Read the model definition and answer for the solid it produces. Units are mm, in the model's axes. Face numbers are marked on the shaded views. A direction names the side the tool comes from. Give positions to 0.01 mm unless a question says otherwise; leave off trailing zeros. Loops run counter-clockwise (first coordinate to the right, second up) from the corner with the lowest first, then second, coordinate; pieces in that order, holes last.
(1) Find section C-C, the plane x = 64.5. Write down the section's boundary in (y, z).
(2) Find section D-D, the plane z = -62.5. Write down the section's boundary in (x, y), then the cut area to 3 significant figures.
(3) Which of the six approach directions +Z, -Z, +X, -X, +Y, -Y give full straight-line access (tool end or side, diameter ignored) to the marked faces 1, 2 and 3?
(4) Find section B-B, the plane z = -46.56. Write down the section's boundary in (x, y), then the cut area to 3 significant figures.
(5) Find section A-A, the plane x = 13.54. Write down the section's boundary in (y, z).
(6) Straight lines are drawn through the part: probe 1 along Z at (x, y) = (128.95, 3.4); probe 2 along Z at (x, y) = (134.03, 3.3); probe 3 along X at (y, z) = (18.25, -23.5). For each, find the intervals that lie inside material, in ascending order.
(7) Each of these flat-tipped pins is pushed along its axis until it touches: P1, Ø7, axis at x = 113.71, z = -66.88, coming from the +Y side; P2, Ø10, axis at x = 36.5, y = 21, coming from the -Z side; P3, Ø7.5, axis at y = 18.5, z = -40.5, coming from the +X side. Where does it stop, or does it pass through?
(8) Determine the mould class of the marked faces 4, 5 and 6 for opening direction Z: pulls with the +Z half, pulls with the -Z half, needs draft (parallel to the pull), parting line crosses it, or undercut.
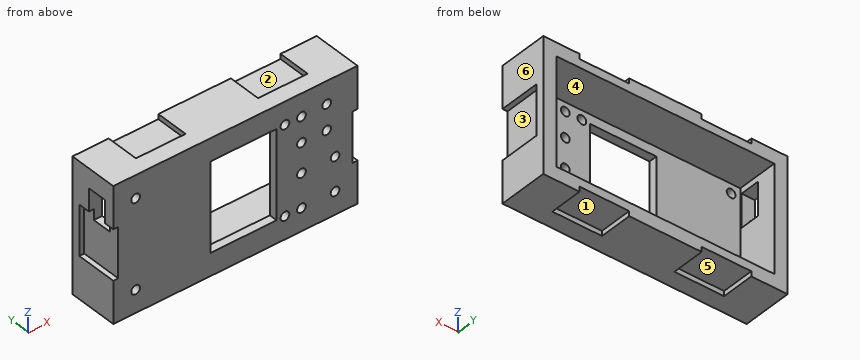
```python
from build123d import *

# Parameters (mm, degrees)
SKETCH1_W                  = 147.57
SKETCH1_H                  = 80.42
BOSS_EXTRUDE1_DEPTH        = 30
SKETCH2_W                  = 131.57
SKETCH2_H                  = 64.42
CUT_EXTRUDE1_DEPTH         = 25
F_4_0_209_DIAMETER_HOLE1_D = 5.3086
SKETCH13_W                 = 30
SKETCH13_H                 = 20
CUT_EXTRUDE3_DEPTH         = 3
MIRROR3_COPY_1_SKETCH_W    = 30
MIRROR3_COPY_1_SKETCH_H    = 20
MIRROR3_COPY_1_DEPTH       = 3
SKETCH19_W                 = 30
SKETCH19_H                 = 25
CUT_EXTRUDE4_DEPTH         = 3
SKETCH25_W                 = 40
SKETCH25_H                 = 53.34
CUT_EXTRUDE5_DEPTH         = 170.909626861
SKETCH30_W                 = 20
SKETCH30_H                 = 12
CUT_EXTRUDE7_DEPTH         = 164.851033869


with BuildPart() as part:
    # Sketch1 → Boss-Extrude1 (new body)
    with BuildSketch(Plane(origin=(0, 0, 0), x_dir=(1, 0, 0), z_dir=(0, 1, 0))):
        with Locations((73.785, 40.21)):
            Rectangle(SKETCH1_W, SKETCH1_H)
    extrude(amount=BOSS_EXTRUDE1_DEPTH)

    # Sketch2 → Cut-Extrude1 (cut)
    with BuildSketch(Plane(origin=(0, 30, 0), x_dir=(1, 0, 0), z_dir=(0, 1, 0))):
        with Locations((73.785, 40.21)):
            Rectangle(SKETCH2_W, SKETCH2_H)
    extrude(amount=-CUT_EXTRUDE1_DEPTH, mode=Mode.SUBTRACT)

    # #4 (0.209) Diameter Hole1 (through all)
    with Locations(Plane(origin=(13.54, 5, -66.88), x_dir=(0, 0, 1), z_dir=(0, 1, 0))):
        with Locations((0, 0), (53.34, 0), (53.34, 90.17), (53.34, 100.17), (38.1, 100.17), (38.1, 115.41), (53.34, 115.41), (20.32, 120.49), (0, 120.49), (0, 100.17), (20.32, 100.17), (0, 90.17)):
            Hole(F_4_0_209_DIAMETER_HOLE1_D / 2)

    # Sketch13 → Cut-Extrude3 (cut)
    with BuildSketch(Plane(origin=(0, 0, -80.42), x_dir=(-1, 0, 0), z_dir=(0, 0, -1))):
        with Locations((-110.6775, 20)):
            Rectangle(SKETCH13_W, SKETCH13_H)
    cut_extrude3 = extrude(amount=-CUT_EXTRUDE3_DEPTH, mode=Mode.SUBTRACT)

    # Mirror2: Cut-Extrude3 across plane
    add(cut_extrude3.mirror(Plane(origin=(73.785, 0, 0), x_dir=(0, 0, 1), z_dir=(1, 0, 0))), mode=Mode.SUBTRACT)

    # Mirror3: Cut-Extrude3 across plane
    add(cut_extrude3.mirror(Plane(origin=(0, 0, -40.21), x_dir=(1, 0, 0), z_dir=(0, 0, -1))), mode=Mode.SUBTRACT)

    # Mirror3 copy 1 sketch → Mirror3 copy 1 (cut)
    with BuildSketch(Plane(origin=(147.57, 0, 0), x_dir=(1, 0, 0), z_dir=(0, 0, 1))):
        with Locations((-110.6775, 20)):
            Rectangle(MIRROR3_COPY_1_SKETCH_W, MIRROR3_COPY_1_SKETCH_H)
    extrude(amount=-MIRROR3_COPY_1_DEPTH, mode=Mode.SUBTRACT)

    # Sketch19 → Cut-Extrude4 (cut)
    with BuildSketch(Plane.ZY):
        with Locations((-40.21, 12.5)):
            Rectangle(SKETCH19_W, SKETCH19_H)
    cut_extrude4 = extrude(amount=-CUT_EXTRUDE4_DEPTH, mode=Mode.SUBTRACT)

    # Mirror7: Cut-Extrude4 across plane
    add(cut_extrude4.mirror(Plane(origin=(73.785, 0, 0), x_dir=(0, 0, 1), z_dir=(1, 0, 0))), mode=Mode.SUBTRACT)

    # Sketch25 → Cut-Extrude5 (cut, through all)
    with BuildSketch(Plane(origin=(0, 5, 0), x_dir=(1, 0, 0), z_dir=(0, 1, 0))):
        with Locations((78.71, 40.21)):
            Rectangle(SKETCH25_W, SKETCH25_H)
    extrude(amount=-CUT_EXTRUDE5_DEPTH, mode=Mode.SUBTRACT)

    # Sketch30 → Cut-Extrude7 (cut, through all)
    with BuildSketch(Plane(origin=(8, 0, 0), x_dir=(0, 0, -1), z_dir=(1, 0, 0))):
        with Locations((21.605, 12)):
            Rectangle(SKETCH30_W, SKETCH30_H)
    extrude(amount=-CUT_EXTRUDE7_DEPTH, mode=Mode.SUBTRACT)


solid = part.part
```
Entries:
1. outline: (0, -80.42) - (30, -80.42) - (30, -72.42) - (5, -72.42) - (5, -66.88) - (0, -66.88) - close; (0, -13.54) - (5, -13.54) - (5, -8) - (30, -8) - (30, 0) - (0, 0) - close
2. outline: (0, 0) - (58.71, 0) - (58.71, 5) - (8, 5) - (8, 30) - (0, 30) - close; (98.71, 0) - (147.57, 0) - (147.57, 30) - (139.57, 30) - (139.57, 5) - (98.71, 5) - close
2. area: 938 mm2
3. face 1: -Z, +Y
3. face 2: +Z, +Y
3. face 3: +X, -Y
4. outline: (0, 25) - (3, 25) - (3, 0) - (58.71, 0) - (58.71, 5) - (8, 5) - (8, 30) - (0, 30) - close; (98.71, 0) - (111.06, 0) - (111.06, 5) - (98.71, 5) - close; (116.36, 0) - (131.38, 0) - (131.38, 5) - (116.36, 5) - close; (136.68, 0) - (144.57, 0) - (144.57, 25) - (147.57, 25) - (147.57, 30) - (139.57, 30) - (139.57, 5) - (136.68, 5) - close
4. area: 735 mm2
5. outline: (0, -80.42) - (30, -80.42) - (30, -72.42) - (5, -72.42) - (5, -69.53) - (0, -69.53) - close; (0, -64.23) - (5, -64.23) - (5, -16.19) - (0, -16.19) - close; (0, -10.89) - (5, -10.89) - (5, -8) - (30, -8) - (30, 0) - (0, 0) - close
6. probe 1: z = -80.42 to -31.43, -26.13 to -16.19, -10.89 to 0
6. probe 2: z = -80.42 to -69.53, -64.23 to -49.21, -43.91 to 0
6. probe 3: x = 0 to 8, 139.57 to 147.57
7. P1: stops at y = 5
7. P2: stops at z = -77.42
7. P3: stops at x = 144.57
8. face 4: undercut
8. face 5: pulls with the -Z half
8. face 6: needs draft
